```python
from build123d import *

# Parameters (mm, degrees)
SKETCH2_R                   = 97.278
SKETCH2_R_2                 = 70.278
BOSS_EXTRUDE2_DEPTH         = 120
SKETCH4_W                   = 7.62
SKETCH4_H                   = 4.2926
CHAMFER1_SIZE               = 3.8
F_1_4_20_TAPPED_HOLE1_D     = 5.1054
F_1_4_20_TAPPED_HOLE1_DEPTH = 25.4
F_1_4_20_TAPPED_HOLE1_TIP   = 1.533816902
F_1_4_20_TAPPED_HOLE2_D     = 5.1054
F_1_4_20_TAPPED_HOLE2_DEPTH = 25.4
F_1_4_20_TAPPED_HOLE2_TIP   = 1.533816902
FILLET1_R                   = 2


with BuildPart() as part:
    # Sketch2 → Boss-Extrude2 (new body)
    with BuildSketch(Plane(origin=(0, 0, 0), x_dir=(1, 0, 0), z_dir=(0, 1, 0))):
        Circle(SKETCH2_R)
        Circle(SKETCH2_R_2, mode=Mode.SUBTRACT)
    extrude(amount=BOSS_EXTRUDE2_DEPTH)

    # Sketch4 → Cut-Revolve1 (revolve, cut)
    with BuildSketch(Plane(origin=(0, 0, 0), x_dir=(0, 0, -1), z_dir=(1, 0, 0))):
        with Locations((89.281, 2.1463)):
            Rectangle(SKETCH4_W, SKETCH4_H)
    revolve(axis=Axis((0, 0, 0), (0, 1, 0)), mode=Mode.SUBTRACT)

    # Chamfer1
    chamfer1_edges = [part.edges().sort_by_distance(p)[0] for p in [
        (-70.278, 120, 0),
    ]]
    chamfer(chamfer1_edges, length=CHAMFER1_SIZE)

    # 1/4-20 Tapped Hole1
    with Locations(Plane(origin=(0, 0, 0), x_dir=(-1, 0, 0), z_dir=(0, -1, 0))):
        with Locations((0, 78.278), (-39.139, 67.790736557), (-67.790736557, 39.139), (-78.278, 0), (-67.790736557, -39.139), (-39.139, -67.790736557), (0, -78.278), (39.139, -67.790736557), (67.790736557, -39.139), (78.278, 0), (67.790736557, 39.139), (39.139, 67.790736557)):
            Hole(F_1_4_20_TAPPED_HOLE1_D / 2, depth=F_1_4_20_TAPPED_HOLE1_DEPTH)
            with Locations((0, 0, -(F_1_4_20_TAPPED_HOLE1_DEPTH + F_1_4_20_TAPPED_HOLE1_TIP / 2))):  # 118° drill point
                Cone(0, F_1_4_20_TAPPED_HOLE1_D / 2, F_1_4_20_TAPPED_HOLE1_TIP, mode=Mode.SUBTRACT)

    # 1/4-20 Tapped Hole2
    with Locations(Plane(origin=(0, 120, 0), x_dir=(1, 0, 0), z_dir=(0, 1, 0))):
        with Locations((-41.25, -71.447095812), (-71.447095812, -41.25), (-82.5, 0), (-71.447095812, 41.25), (-41.25, 71.447095812), (0, 82.5), (41.25, 71.447095812), (71.447095812, 41.25), (82.5, 0), (71.447095812, -41.25), (41.25, -71.447095812), (0, -82.5)):
            Hole(F_1_4_20_TAPPED_HOLE2_D / 2, depth=F_1_4_20_TAPPED_HOLE2_DEPTH)
            with Locations((0, 0, -(F_1_4_20_TAPPED_HOLE2_DEPTH + F_1_4_20_TAPPED_HOLE2_TIP / 2))):  # 118° drill point
                Cone(0, F_1_4_20_TAPPED_HOLE2_D / 2, F_1_4_20_TAPPED_HOLE2_TIP, mode=Mode.SUBTRACT)

    # Fillet1
    fillet1_edges = [part.edges().sort_by_distance(p)[0] for p in [
        (-97.278, 120, 0),
    ]]
    fillet(fillet1_edges, radius=FILLET1_R)


solid = part.part
```
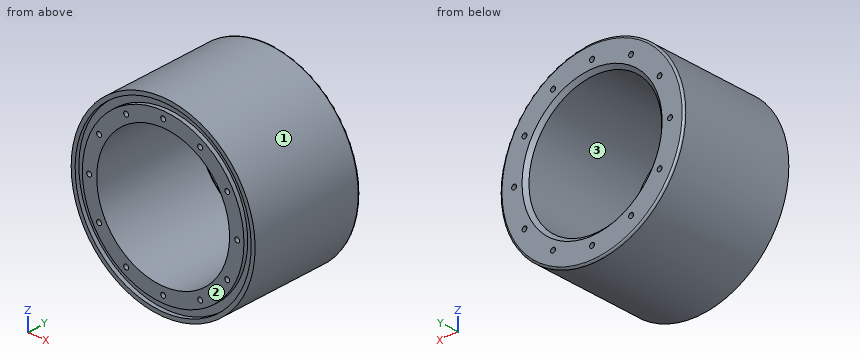
Here's how the part is built. I have some questions about the finished solid (model axes, mm). Face numbers are marked on the shaded views. Round coordinates to 2 decimals unless told otherwise and drop trailing zeros. Write each loop counter-clockwise with the first axis right and the second up, starting at its lowest first coordinate (ties: lowest second). Pieces come first, ordered by that corner, then holes.
Q1. Please list where these lines run through material, in increasing order: probe 1 along X at (y, z) = (96, -42); probe 2 along X at (y, z) = (104, 41.25); probe 3 along X at (y, z) = (114.5, 71).
Q2. Will these pins go through, and if not, where does the flat tip stop? P1, Ø4, axis at x = -64.5, y = 53.5, coming from the +Z side; P2, Ø1, axis at y = 12, z = 59.5, coming from the +X side; P3, Ø1, axis at x = 49.5, y = 59.5, coming from the +Z side.
Q3. If we mould it in two halves opening along Z, with no side actions, what happens to the marked faces 1, 2 and 3? For each: +Z half, -Z half, draft (parallel to the pull), parting line (faces both ways), or undercut.
Q4. If we section it at A-A on y = 14: Give the number of separate pieces and of enclosed holes in the cut face, plus the area to 3 significant figures.
Q5. If we section it at B-B on y = 34.5: Write out the boundary of the cut face in (x, z).
Answer below:
1. probe 1: x = -87.74 to -73.89, -69.01 to -56.35, 56.35 to 69.01, 73.89 to 87.74
1. probe 2: x = -88.1 to -74, -68.89 to -56.9, 56.9 to 68.89, 74 to 88.1
1. probe 3: x = -66.5 to -43.76, -38.74 to 38.74, 43.76 to 66.5
2. P1: stops at z = 74.54
2. P2: stops at x = 77.34
2. P3: stops at z = 84.04
3. face 1: parting line
3. face 2: draft
3. face 3: undercut
4. separate pieces: 1
4. enclosed holes: 13
4. area: 14,000 mm2
5. outline: circle Ø194.56 at (0, 0); hole circle Ø140.56 at (0, 0)
